```python
from build123d import *

# Parameters (mm, degrees)
SKETCH_1_W          = 40
SKETCH_1_H          = 40
SKETCH_1_W_2        = 30
SKETCH_1_H_2        = 15
EXTRUDE_1_DEPTH     = 50
CUT_EXTRUDE_START   = -50
SKETCH_3_W          = 28
SKETCH_3_H          = 25
CUT_EXTRUDE_1_DEPTH = 50
CHAMFER_1_SIZE      = 1
CUT_EXTRUDE_2_REACH = 77.498
SKETCH_4_R          = 1.75
SKETCH_5_W          = 2
SKETCH_5_H          = 10
CUT_EXTRUDE_4_DEPTH = 76.498344353
CHAMFER_3_SIZE      = 1


with BuildPart() as part:
    # ｽｹｯﾁ1 → ﾎﾞｽ - 押し出し1 (new body)
    with BuildSketch(Plane.XY):
        with Locations((20, 20)):
            Rectangle(SKETCH_1_W, SKETCH_1_H)
        with Locations((20, 12.5)):
            Rectangle(SKETCH_1_W_2, SKETCH_1_H_2, mode=Mode.SUBTRACT)
    extrude(amount=EXTRUDE_1_DEPTH)

    # ｽｹｯﾁ3 → ｶｯﾄ - 押し出し1 (cut)
    with BuildSketch(Plane(origin=(0, 0, 0), x_dir=(-1, 0, 0), z_dir=(0, 0, -1)).offset(CUT_EXTRUDE_START)):
        with Locations((-20, 12.5)):
            Rectangle(SKETCH_3_W, SKETCH_3_H)
    extrude(amount=CUT_EXTRUDE_1_DEPTH, mode=Mode.SUBTRACT)

    # 面取り1
    chamfer_1_edges = [part.edges().sort_by_distance(p)[0] for p in [
        (6, 20, 25),
        (6, 5, 25),
        (34, 5, 25),
        (34, 20, 25),
    ]]
    chamfer(chamfer_1_edges, length=CHAMFER_1_SIZE - 0.0001)  # a hair under: the kernel refuses the full size

    # ｽｹｯﾁ4 → ｶｯﾄ - 押し出し2 (cut, up to next)
    with BuildSketch(Plane(origin=(0, 40, 0), x_dir=(1, 0, 0), z_dir=(0, 1, 0)), mode=Mode.PRIVATE) as cut_extrude_2_sk1:
        with Locations(Location((10, -5, 0), (0, 0, 270))):
            Circle(SKETCH_4_R)
    cut_extrude_2_tool1 = extrude(cut_extrude_2_sk1.sketch, amount=-CUT_EXTRUDE_2_REACH, mode=Mode.PRIVATE) & part.part
    # ｽｹｯﾁ4 → ｶｯﾄ - 押し出し2 (cut, up to next)
    with BuildSketch(Plane(origin=(0, 40, 0), x_dir=(1, 0, 0), z_dir=(0, 1, 0)), mode=Mode.PRIVATE) as cut_extrude_2_sk2:
        with Locations(Location((20, -5, 0), (0, 0, 270))):
            Circle(SKETCH_4_R)
    cut_extrude_2_tool2 = extrude(cut_extrude_2_sk2.sketch, amount=-CUT_EXTRUDE_2_REACH, mode=Mode.PRIVATE) & part.part
    # ｽｹｯﾁ4 → ｶｯﾄ - 押し出し2 (cut, up to next)
    with BuildSketch(Plane(origin=(0, 40, 0), x_dir=(1, 0, 0), z_dir=(0, 1, 0)), mode=Mode.PRIVATE) as cut_extrude_2_sk3:
        with Locations(Location((30, -5, 0), (0, 0, 270))):
            Circle(SKETCH_4_R)
    cut_extrude_2_tool3 = extrude(cut_extrude_2_sk3.sketch, amount=-CUT_EXTRUDE_2_REACH, mode=Mode.PRIVATE) & part.part
    # ｽｹｯﾁ4 → ｶｯﾄ - 押し出し2 (cut, up to next)
    with BuildSketch(Plane(origin=(0, 40, 0), x_dir=(1, 0, 0), z_dir=(0, 1, 0)), mode=Mode.PRIVATE) as cut_extrude_2_sk4:
        with Locations(Location((10, -15, 0), (0, 0, 270))):
            Circle(SKETCH_4_R)
    cut_extrude_2_tool4 = extrude(cut_extrude_2_sk4.sketch, amount=-CUT_EXTRUDE_2_REACH, mode=Mode.PRIVATE) & part.part
    # ｽｹｯﾁ4 → ｶｯﾄ - 押し出し2 (cut, up to next)
    with BuildSketch(Plane(origin=(0, 40, 0), x_dir=(1, 0, 0), z_dir=(0, 1, 0)), mode=Mode.PRIVATE) as cut_extrude_2_sk5:
        with Locations(Location((20, -15, 0), (0, 0, 270))):
            Circle(SKETCH_4_R)
    cut_extrude_2_tool5 = extrude(cut_extrude_2_sk5.sketch, amount=-CUT_EXTRUDE_2_REACH, mode=Mode.PRIVATE) & part.part
    # ｽｹｯﾁ4 → ｶｯﾄ - 押し出し2 (cut, up to next)
    with BuildSketch(Plane(origin=(0, 40, 0), x_dir=(1, 0, 0), z_dir=(0, 1, 0)), mode=Mode.PRIVATE) as cut_extrude_2_sk6:
        with Locations(Location((30, -15, 0), (0, 0, 270))):
            Circle(SKETCH_4_R)
    cut_extrude_2_tool6 = extrude(cut_extrude_2_sk6.sketch, amount=-CUT_EXTRUDE_2_REACH, mode=Mode.PRIVATE) & part.part
    # ｽｹｯﾁ4 → ｶｯﾄ - 押し出し2 (cut, up to next)
    with BuildSketch(Plane(origin=(0, 40, 0), x_dir=(1, 0, 0), z_dir=(0, 1, 0)), mode=Mode.PRIVATE) as cut_extrude_2_sk7:
        with Locations(Location((10, -25, 0), (0, 0, 270))):
            Circle(SKETCH_4_R)
    cut_extrude_2_tool7 = extrude(cut_extrude_2_sk7.sketch, amount=-CUT_EXTRUDE_2_REACH, mode=Mode.PRIVATE) & part.part
    # ｽｹｯﾁ4 → ｶｯﾄ - 押し出し2 (cut, up to next)
    with BuildSketch(Plane(origin=(0, 40, 0), x_dir=(1, 0, 0), z_dir=(0, 1, 0)), mode=Mode.PRIVATE) as cut_extrude_2_sk8:
        with Locations(Location((20, -25, 0), (0, 0, 270))):
            Circle(SKETCH_4_R)
    cut_extrude_2_tool8 = extrude(cut_extrude_2_sk8.sketch, amount=-CUT_EXTRUDE_2_REACH, mode=Mode.PRIVATE) & part.part
    # ｽｹｯﾁ4 → ｶｯﾄ - 押し出し2 (cut, up to next)
    with BuildSketch(Plane(origin=(0, 40, 0), x_dir=(1, 0, 0), z_dir=(0, 1, 0)), mode=Mode.PRIVATE) as cut_extrude_2_sk9:
        with Locations(Location((30, -25, 0), (0, 0, 270))):
            Circle(SKETCH_4_R)
    cut_extrude_2_tool9 = extrude(cut_extrude_2_sk9.sketch, amount=-CUT_EXTRUDE_2_REACH, mode=Mode.PRIVATE) & part.part
    # ｽｹｯﾁ4 → ｶｯﾄ - 押し出し2 (cut, up to next)
    with BuildSketch(Plane(origin=(0, 40, 0), x_dir=(1, 0, 0), z_dir=(0, 1, 0)), mode=Mode.PRIVATE) as cut_extrude_2_sk10:
        with Locations(Location((10, -35, 0), (0, 0, 270))):
            Circle(SKETCH_4_R)
    cut_extrude_2_tool10 = extrude(cut_extrude_2_sk10.sketch, amount=-CUT_EXTRUDE_2_REACH, mode=Mode.PRIVATE) & part.part
    # ｽｹｯﾁ4 → ｶｯﾄ - 押し出し2 (cut, up to next)
    with BuildSketch(Plane(origin=(0, 40, 0), x_dir=(1, 0, 0), z_dir=(0, 1, 0)), mode=Mode.PRIVATE) as cut_extrude_2_sk11:
        with Locations(Location((20, -35, 0), (0, 0, 270))):
            Circle(SKETCH_4_R)
    cut_extrude_2_tool11 = extrude(cut_extrude_2_sk11.sketch, amount=-CUT_EXTRUDE_2_REACH, mode=Mode.PRIVATE) & part.part
    # ｽｹｯﾁ4 → ｶｯﾄ - 押し出し2 (cut, up to next)
    with BuildSketch(Plane(origin=(0, 40, 0), x_dir=(1, 0, 0), z_dir=(0, 1, 0)), mode=Mode.PRIVATE) as cut_extrude_2_sk12:
        with Locations(Location((30, -35, 0), (0, 0, 270))):
            Circle(SKETCH_4_R)
    cut_extrude_2_tool12 = extrude(cut_extrude_2_sk12.sketch, amount=-CUT_EXTRUDE_2_REACH, mode=Mode.PRIVATE) & part.part
    # ｽｹｯﾁ4 → ｶｯﾄ - 押し出し2 (cut, up to next)
    with BuildSketch(Plane(origin=(0, 40, 0), x_dir=(1, 0, 0), z_dir=(0, 1, 0)), mode=Mode.PRIVATE) as cut_extrude_2_sk13:
        with Locations(Location((10, -45, 0), (0, 0, 270))):
            Circle(SKETCH_4_R)
    cut_extrude_2_tool13 = extrude(cut_extrude_2_sk13.sketch, amount=-CUT_EXTRUDE_2_REACH, mode=Mode.PRIVATE) & part.part
    # ｽｹｯﾁ4 → ｶｯﾄ - 押し出し2 (cut, up to next)
    with BuildSketch(Plane(origin=(0, 40, 0), x_dir=(1, 0, 0), z_dir=(0, 1, 0)), mode=Mode.PRIVATE) as cut_extrude_2_sk14:
        with Locations(Location((20, -45, 0), (0, 0, 270))):
            Circle(SKETCH_4_R)
    cut_extrude_2_tool14 = extrude(cut_extrude_2_sk14.sketch, amount=-CUT_EXTRUDE_2_REACH, mode=Mode.PRIVATE) & part.part
    # ｽｹｯﾁ4 → ｶｯﾄ - 押し出し2 (cut, up to next)
    with BuildSketch(Plane(origin=(0, 40, 0), x_dir=(1, 0, 0), z_dir=(0, 1, 0)), mode=Mode.PRIVATE) as cut_extrude_2_sk15:
        with Locations(Location((30, -45, 0), (0, 0, 270))):
            Circle(SKETCH_4_R)
    cut_extrude_2_tool15 = extrude(cut_extrude_2_sk15.sketch, amount=-CUT_EXTRUDE_2_REACH, mode=Mode.PRIVATE) & part.part
    add(cut_extrude_2_tool1.solids().sort_by_distance((10, 40, 5))[0], mode=Mode.SUBTRACT)
    add(cut_extrude_2_tool2.solids().sort_by_distance((20, 40, 5))[0], mode=Mode.SUBTRACT)
    add(cut_extrude_2_tool3.solids().sort_by_distance((30, 40, 5))[0], mode=Mode.SUBTRACT)
    add(cut_extrude_2_tool4.solids().sort_by_distance((10, 40, 15))[0], mode=Mode.SUBTRACT)
    add(cut_extrude_2_tool5.solids().sort_by_distance((20, 40, 15))[0], mode=Mode.SUBTRACT)
    add(cut_extrude_2_tool6.solids().sort_by_distance((30, 40, 15))[0], mode=Mode.SUBTRACT)
    add(cut_extrude_2_tool7.solids().sort_by_distance((10, 40, 25))[0], mode=Mode.SUBTRACT)
    add(cut_extrude_2_tool8.solids().sort_by_distance((20, 40, 25))[0], mode=Mode.SUBTRACT)
    add(cut_extrude_2_tool9.solids().sort_by_distance((30, 40, 25))[0], mode=Mode.SUBTRACT)
    add(cut_extrude_2_tool10.solids().sort_by_distance((10, 40, 35))[0], mode=Mode.SUBTRACT)
    add(cut_extrude_2_tool11.solids().sort_by_distance((20, 40, 35))[0], mode=Mode.SUBTRACT)
    add(cut_extrude_2_tool12.solids().sort_by_distance((30, 40, 35))[0], mode=Mode.SUBTRACT)
    add(cut_extrude_2_tool13.solids().sort_by_distance((10, 40, 45))[0], mode=Mode.SUBTRACT)
    add(cut_extrude_2_tool14.solids().sort_by_distance((20, 40, 45))[0], mode=Mode.SUBTRACT)
    add(cut_extrude_2_tool15.solids().sort_by_distance((30, 40, 45))[0], mode=Mode.SUBTRACT)

    # ｽｹｯﾁ5 → ｶｯﾄ - 押し出し4 (cut, through all)
    with BuildSketch(Plane(origin=(40, 0, 0), x_dir=(0, 0, -1), z_dir=(1, 0, 0))):
        with Locations((-5, 12.5)):
            Rectangle(SKETCH_5_W, SKETCH_5_H)
    extrude(amount=-CUT_EXTRUDE_4_DEPTH, mode=Mode.SUBTRACT)

    # 面取り3
    chamfer_3_edges = [part.edges().sort_by_distance(p)[0] for p in [
        (2.5, 17.5, 6),
        (2.5, 17.5, 4),
        (2.5, 7.5, 4),
        (2.5, 7.5, 6),
        (37.5, 7.5, 4),
        (37.5, 7.5, 6),
        (37.5, 17.5, 4),
        (37.5, 17.5, 6),
    ]]
    chamfer(chamfer_3_edges, length=CHAMFER_3_SIZE - 0.0001)  # a hair under: the kernel refuses the full size


solid = part.part
```
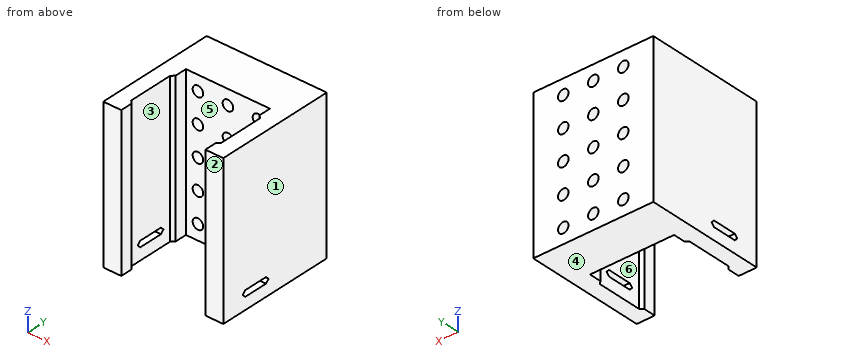
The model under review builds one solid part; all positions refer to its coordinate system, in mm. Face numbers are marked on the shaded views. A direction names the side the tool comes from. Round coordinates to 2 decimals unless told otherwise and drop trailing zeros. Loops run counter-clockwise (first coordinate to the right, second up) from the corner with the lowest first, then second, coordinate; pieces in that order, holes last. Notation, with made-up numbers: (85, -31.75) -> (117, -31.75) arc R33 cw to (117, 2.25) -> close; hole circle Ø6 at (-30.5, -22.5). An arc over 180 degrees is marked (long way). Answer as a JSON object with one key per item and string values. Group by question number.
1) For the marked faces 4, 5 and 6, list the 3-axis set-ups (+Z, -Z, +X, -X, +Y, -Y) from which the entire face can be reached by the end or side of a thin tool; tool diameter is ignored.
2) We need section C-C on z = 25. Give the number of separate pieces and of enclosed holes in the cut face, then the cut area to 4 significant figures.
3) For line 1 (X direction, y = 36, z = 25); line 2 (X direction, y = 7, z = 30); line 3 (X direction, y = 21, z = 31.5), list the stretches that pass through material, from the lowest coordinate up. Write a range as [from, to].
4) We need section B-B on y = 6.5. Write out the cut boundary in (x, z).
5) For pin 1 Ø4 at (x, z) = (14, 44.5) entering from -Y, flat-tipped, find the tip position at first contact; note if it passes through.
6) We need section A-A on x = 30. Write out the cut boundary in (y, z).
7) Mouldability with a two-part tool opening along Y and no side actions: class the marked faces 1, 2 and 3 as released by +Y, released by -Y, zero draft, split by the parting line, or undercut.
Result set:
{
 "1": {"face 4": "-Z, +X, -X, +Y, -Y", "face 5": "+Z, -Z, -Y", "face 6": "+Z, -Z"},
 "2": {"separate pieces": "4", "enclosed holes": "0", "area": "710.5 mm²"},
 "3": {"line 1": "[0, 8.25], [11.75, 18.25], [21.75, 28.25], [31.75, 40]", "line 2": "[0, 5], [35, 40]", "line 3": "[0, 6], [34, 40]"},
 "4": {"outline": "(0, 0) -> (5, 0) -> (5, 50) -> (0, 50) -> close; (35, 0) -> (40, 0) -> (40, 50) -> (35, 50) -> close"},
 "5": {"pin 1": "y = 25"},
 "6": {"outline": "(25, 0) -> (40, 0) -> (40, 3.25) -> (25, 3.25) -> close; (25, 6.75) -> (40, 6.75) -> (40, 13.25) -> (25, 13.25) -> close; (25, 16.75) -> (40, 16.75) -> (40, 23.25) -> (25, 23.25) -> close; (25, 26.75) -> (40, 26.75) -> (40, 33.25) -> (25, 33.25) -> close; (25, 36.75) -> (40, 36.75) -> (40, 43.25) -> (25, 43.25) -> close; (25, 46.75) -> (40, 46.75) -> (40, 50) -> (25, 50) -> close"},
 "7": {"face 1": "zero draft", "face 2": "released by -Y", "face 3": "undercut"}
}
